Design review of the part built by this model. Coordinates are the model's own, in mm. Face numbers are marked on the shaded views. A direction names the side the tool comes from. Give positions to 0.01 mm unless a question says otherwise; leave off trailing zeros. Loops run counter-clockwise (first coordinate to the right, second up) from the corner with the lowest first, then second, coordinate; pieces in that order, holes last. Notation, with made-up numbers: (-24, -31.5) -> (23, -31.5) arc R23 ccw to (23, -5.5) -> close; hole circle Ø11 at (-19.75, 50). An arc over 180 degrees is marked (long way). Use a Markdown table: item, result. Add a question column.
1. For the marked faces 1, 2 and 3, list the 3-axis set-ups (+Z, -Z, +X, -X, +Y, -Y) from which the entire face can be reached by the end or side of a thin tool; tool diameter is ignored.
2. Draft analysis for pull direction Y (two halves, no side actions). For the marked faces 4, 5 and 6, state which applies: pulls with the +Y half, pulls with the -Y half, needs draft (parallel to the pull), parting line crosses it, or undercut.
3. To check wall thickness, follow line 1 (X direction, y = 3.5, z = 8.5); line 2 (Z direction, x = 5.25, y = 8) (1 decimal); line 3 (X direction, y = 10, z = 1.25). State the ranges of each line that lie inside material, in increasing order.
4. Add section C-C (x = -3.75). State the section outline as (y, z) points.
5. Add section A-A (y = -18.35). State the section outline as (x, z) points, and give its area (3 significant figures).
6. For pin 1 Ø1.6 at (x, z) = (4, 1) entering from +Y; pin 2 Ø1.5 at (x, z) = (4, 2) entering from +Y; pin 3 Ø2.5 at (x, z) = (-0.5, 1) entering from -Y; pin 4 Ø3 at (y, z) = (-13.5, 10) entering from +X, all flat-tipped, find the tip position at first contact; note any pin that passes through.
7. Add section D-D (y = -4). State the section outline as (x, z) points (1 decimal).
8. Add section B-B (x = 0.5). Count the separate pieces of the cut face and the enclosed holes in it, and give its area (3 significant figures).
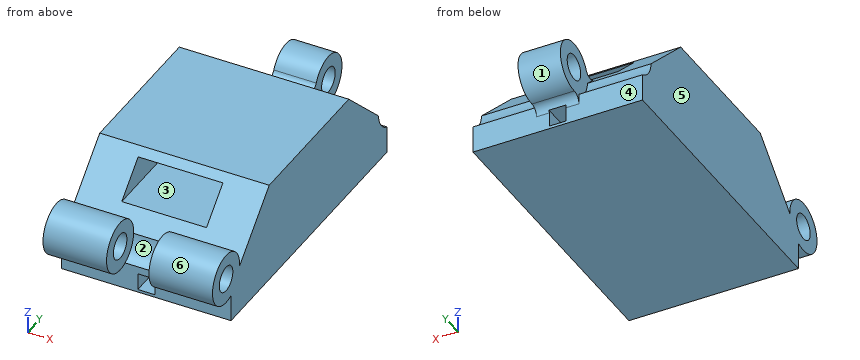
```python
from build123d import *

# Parameters (mm, degrees)
SKETCH2_W                       = 20
SKETCH2_H                       = 34.5
BOSS_EXTRUDE1_DEPTH             = 15
CUT_EXTRUDE1_DEPTH              = 25.951202376
CUT_EXTRUDE1_DEPTH_BACK         = 25.951202376
CUT_EXTRUDE2_DEPTH              = 25.951202376
CUT_EXTRUDE2_DEPTH_BACK         = 25.951202376
CUT_EXTRUDE4_DEPTH              = 25.951202376
CUT_EXTRUDE4_DEPTH_BACK         = 25.951202376
SKETCH10_R                      = 3
SKETCH12_R                      = 3
SKETCH12_R_2                    = 1.5
BOSS_EXTRUDE4_DEPTH             = 2.5
FILLET4_R                       = 1
BOSS_EXTRUDE5_REACH             = 29.943
SKETCH13_R                      = 3
SKETCH13_R_2                    = 1.5
BOSS_EXTRUDE5_DIRECTION_2_REACH = 29.943
SKETCH14_R                      = 3
CUT_EXTRUDE6_DEPTH              = 2.5
CUT_EXTRUDE7_DEPTH              = 28.94320132
CUT_EXTRUDE7_DEPTH_BACK         = 28.94320132
CUT_EXTRUDE8_REACH              = 29.273
SKETCH17_W                      = 10
SKETCH17_H                      = 3.4375
CUT_EXTRUDE8_DIRECTION_2_REACH  = 29.273
SKETCH18_W                      = 2
SKETCH18_H                      = 38.848747282
CUT_EXTRUDE9_DEPTH              = 1


with BuildPart() as part:
    # Sketch2 → Boss-Extrude1 (new body)
    with BuildSketch(Plane.XY):
        with Locations((2, 0)):
            Rectangle(SKETCH2_W, SKETCH2_H)
    extrude(amount=BOSS_EXTRUDE1_DEPTH)

    # Sketch6 → Cut-Extrude1 (cut, two sides: drawn at the far end of the back side and taken through both)
    with BuildSketch(Plane(origin=(2, 0, 0), x_dir=(0, 0, -1), z_dir=(1, 0, 0)).offset(-CUT_EXTRUDE1_DEPTH_BACK)):
        Polygon((-4, 17.25), (-15, 5.631049961), (-15, 17.25), align=None)
    extrude(amount=CUT_EXTRUDE1_DEPTH + CUT_EXTRUDE1_DEPTH_BACK, mode=Mode.SUBTRACT)

    # Sketch8 → Cut-Extrude2 (cut, two sides: drawn at the far end of the back side and taken through both)
    with BuildSketch(Plane(origin=(2, 0, 0), x_dir=(0, 0, -1), z_dir=(1, 0, 0)).offset(-CUT_EXTRUDE2_DEPTH_BACK)):
        Polygon((-4, -17.25), (-15, -5.631049961), (-15, -17.25), align=None)
    extrude(amount=CUT_EXTRUDE2_DEPTH + CUT_EXTRUDE2_DEPTH_BACK, mode=Mode.SUBTRACT)

    # Sketch10 → Cut-Extrude4 (cut, two sides: drawn at the far end of the back side and taken through both)
    with BuildSketch(Plane(origin=(2, 0, 0), x_dir=(0, 0, -1), z_dir=(1, 0, 0)).offset(-CUT_EXTRUDE4_DEPTH_BACK)):
        with Locations((-6, 18.35)):
            Circle(SKETCH10_R)
    extrude(amount=CUT_EXTRUDE4_DEPTH + CUT_EXTRUDE4_DEPTH_BACK, mode=Mode.SUBTRACT)

    # Sketch12 → Boss-Extrude4 (add, symmetric)
    with BuildSketch(Plane(origin=(2, 0, 0), x_dir=(0, 0, -1), z_dir=(1, 0, 0))):
        with Locations((-6, 18.35)):
            Circle(SKETCH12_R)
        with Locations((-6, 18.35)):
            Circle(SKETCH12_R_2, mode=Mode.SUBTRACT)
    extrude(amount=BOSS_EXTRUDE4_DEPTH, both=True)

    # Fillet4
    fillet4_edges = [part.edges().sort_by_distance(p)[0] for p in [
        (2, 15.357223012, 5.791947362),
        (2, 17.25, 3.208942853),
    ]]
    fillet(fillet4_edges, radius=FILLET4_R)

    # Boss-Extrude5: up to this face of the body (flat: up to its plane)
    boss_extrude5_end = Plane(part.part.faces().sort_by_distance((12, -0.0739089, 6.251251182))[0])
    # Sketch13 → Boss-Extrude5 (add, up to the picked face)
    with BuildSketch(Plane(origin=(2, 0, 0), x_dir=(0, 0, -1), z_dir=(1, 0, 0)), mode=Mode.PRIVATE) as boss_extrude5_sk1:
        with Locations((-6, -18.35)):
            Circle(SKETCH13_R)
        with Locations(Location((-6, -18.35, 0), (0, 0, 180))):
            Circle(SKETCH13_R_2, mode=Mode.SUBTRACT)
    boss_extrude5_tool1 = split(extrude(boss_extrude5_sk1.sketch, amount=BOSS_EXTRUDE5_REACH, mode=Mode.PRIVATE), bisect_by=boss_extrude5_end, keep=Keep.BOTH, mode=Mode.PRIVATE)
    add(boss_extrude5_tool1.solids().sort_by(Axis((2, -18.35, 8.915147), (1, 0, 0)))[0])

    # Boss-Extrude5 direction 2: up to this face of the body (flat: up to its plane)
    boss_extrude5_direction_2_end = Plane(part.part.faces().sort_by_distance((-8, -0.0739089, 6.251251182))[0])
    # Sketch13 → Boss-Extrude5 direction 2 (add, up to the picked face)
    with BuildSketch(Plane(origin=(2, 0, 0), x_dir=(0, 0, -1), z_dir=(1, 0, 0)), mode=Mode.PRIVATE) as boss_extrude5_direction_2_sk1:
        with Locations((-6, -18.35)):
            Circle(SKETCH13_R)
        with Locations(Location((-6, -18.35, 0), (0, 0, 180))):
            Circle(SKETCH13_R_2, mode=Mode.SUBTRACT)
    boss_extrude5_direction_2_tool1 = split(extrude(boss_extrude5_direction_2_sk1.sketch, amount=-BOSS_EXTRUDE5_DIRECTION_2_REACH, mode=Mode.PRIVATE), bisect_by=boss_extrude5_direction_2_end, keep=Keep.BOTH, mode=Mode.PRIVATE)
    add(boss_extrude5_direction_2_tool1.solids().sort_by(Axis((2, -18.35, 8.915147), (-1, 0, 0)))[0])

    # Sketch14 → Cut-Extrude6 (cut, symmetric)
    with BuildSketch(Plane(origin=(2, 0, 0), x_dir=(0, 0, -1), z_dir=(1, 0, 0))):
        with Locations((-6, -18.35)):
            Circle(SKETCH14_R)
    extrude(amount=CUT_EXTRUDE6_DEPTH, both=True, mode=Mode.SUBTRACT)

    # Sketch15 → Cut-Extrude7 (cut, two sides: drawn at the far end of the back side and taken through both)
    with BuildSketch(Plane(origin=(2, 0, 0), x_dir=(0, 0, -1), z_dir=(1, 0, 0)).offset(-CUT_EXTRUDE7_DEPTH_BACK)):
        Polygon((-16.548060764, -12.233536013), (-12, -12.233536013), (-12, 0), (-12, 8.799854517), (-16.548060764, 8.799854517), (-16.548060764, -7.042323617), align=None)
    extrude(amount=CUT_EXTRUDE7_DEPTH + CUT_EXTRUDE7_DEPTH_BACK, mode=Mode.SUBTRACT)

    # Cut-Extrude8: up to this plane
    cut_extrude8_end = Plane(origin=(-8, -17.25, 4), z_dir=(0, 0.6875, -0.7261843774138907))
    # Sketch17 → Cut-Extrude8 (cut, up to the surface)
    with BuildSketch(Plane(origin=(0, 0, 0), x_dir=(1, 0, 0), z_dir=(0, 1, 0)), mode=Mode.PRIVATE) as cut_extrude8_sk1:
        with Locations((2, -9.45625)):
            Rectangle(SKETCH17_W, SKETCH17_H)
    cut_extrude8_tool1 = split(extrude(cut_extrude8_sk1.sketch, amount=-CUT_EXTRUDE8_REACH, mode=Mode.PRIVATE), bisect_by=cut_extrude8_end, keep=Keep.BOTH, mode=Mode.PRIVATE)
    add(cut_extrude8_tool1.solids().sort_by_distance((2, 0, 9.45625))[0], mode=Mode.SUBTRACT)

    # Cut-Extrude8 direction 2: up to this plane
    cut_extrude8_direction_2_end = Plane(origin=(-8, 17.25, 4), z_dir=(0, 0.6875, 0.7261843774138907))
    # Sketch17 → Cut-Extrude8 direction 2 (cut, up to the surface)
    with BuildSketch(Plane(origin=(0, 0, 0), x_dir=(1, 0, 0), z_dir=(0, 1, 0)), mode=Mode.PRIVATE) as cut_extrude8_direction_2_sk1:
        with Locations((2, -9.45625)):
            Rectangle(SKETCH17_W, SKETCH17_H)
    cut_extrude8_direction_2_tool1 = split(extrude(cut_extrude8_direction_2_sk1.sketch, amount=CUT_EXTRUDE8_DIRECTION_2_REACH, mode=Mode.PRIVATE), bisect_by=cut_extrude8_direction_2_end, keep=Keep.BOTH, mode=Mode.PRIVATE)
    add(cut_extrude8_direction_2_tool1.solids().sort_by_distance((2, 0, 9.45625))[0], mode=Mode.SUBTRACT)

    # Sketch18 → Cut-Extrude9 (cut, symmetric)
    with BuildSketch(Plane(origin=(2, 0, 0), x_dir=(0, 0, -1), z_dir=(1, 0, 0))):
        with Locations((-1.32, 2.174373641)):
            Rectangle(SKETCH18_W, SKETCH18_H)
    extrude(amount=CUT_EXTRUDE9_DEPTH, both=True, mode=Mode.SUBTRACT)


solid = part.part
```
Taken from the geometry:
| question | item | result |
|---|---|---|
| 1 | face 1 | +X, -X |
| 1 | face 2 | +Z, -Y |
| 1 | face 3 | none |
| 2 | face 4 | pulls with the +Y half |
| 2 | face 5 | needs draft |
| 2 | face 6 | undercut |
| 3 | line 1 | x = -8 to -3, 7 to 12 |
| 3 | line 2 | z = 0 to 7.7, 11.2 to 12 |
| 3 | line 3 | x = -8 to 1, 3 to 12 |
| 4 | outline | (-17.25, 0) -> (17.25, 0) -> (17.25, 3.21) arc R3 cw to (15.36, 5.79) -> (8.8, 12) -> (-8.8, 12) -> (-15.36, 5.79) arc R3 ccw (long way) to (-17.25, 3.21) -> close; hole circle Ø3 at (-18.35, 6) |
| 5 | outline | (-8, 3) -> (-0.5, 3) -> (-0.5, 4.5) -> (-8, 4.5) -> close; (-8, 7.5) -> (-0.5, 7.5) -> (-0.5, 9) -> (-8, 9) -> close; (4.5, 3) -> (12, 3) -> (12, 4.5) -> (4.5, 4.5) -> close; (4.5, 7.5) -> (12, 7.5) -> (12, 9) -> (4.5, 9) -> close |
| 5 | area | 45.0 mm^2 |
| 6 | pin 1 | stops at y = 17.25 |
| 6 | pin 2 | stops at y = 17.59 |
| 6 | pin 3 | stops at y = -17.25 |
| 6 | pin 4 | passes through |
| 7 | outline | (-8, 0) -> (12, 0) -> (12, 12) -> (-8, 12) -> close; hole (-3, 7.7) -> (7, 7.7) -> (7, 11.2) -> (-3, 11.2) -> close; hole (1, 0.3) -> (3, 0.3) -> (3, 2.3) -> (1, 2.3) -> close |
| 8 | separate pieces | 2 |
| 8 | enclosed holes | 1 |
| 8 | area | 286 mm^2 |
